Autodesk Inventor part; units mm, degrees
ref_plane "YZ Plane" through (0, 0, 0) normal (1, 0, 0) x (0, 1, 0)
ref_plane "XZ Plane" through (0, 0, 0) normal (0, 1, 0) x (-1, 0, 0)
ref_plane "XY Plane" through (0, 0, 0) normal (0, 0, 1) x (1, 0, 0)
sketch "Sketch1" plane through (0, 0, 0) normal (0, 1, 0) x (-1, 0, 0)
  circle A0 centre (0, 0) radius 10.7
  dimension "d0" = 21.4
extrude "Extrusion1" add sketch "Sketch1" along normal blind 19
sketch "Sketch2" plane through (0, 19, 0) normal (0, 1, 0) x (1, 0, 0)
  circle A0 centre (0, 0) radius 12.5
  circle A1 centre (0, 0) radius 10.7
  line L0 (-15, 8) -> (15, 8)
  line L1 (15, 8) -> (15, -8)
  line L2 (15, -8) -> (-15, -8)
  line L3 (-15, -8) -> (-15, 8)
  line L4 (0, 0) -> (1.899, 0)
  line L5 (0, 0) -> (0, 1.5989)
  point P0 (-12.5, 0)
  point P1 (9.6047, -8)
  point P2 (-9.6047, 8)
  point P3 (12.5, 0)
  point P4 (-9.6047, -8)
  point P5 (9.6047, 8)
  dimension "d9" = 25
  dimension "d10" = 21.4
  dimension "d14" = 30
  dimension "d15" = 16
extrude "Extrusion2" add sketch "Sketch2" along normal blind 5
sketch "Sketch3" plane through (0, 0, 0) normal (0, 0, 1) x (1, 0, 0)
  line L0 (10.7, 0) -> (-10.7, 0)
  line L1 (9.6047, 19) -> (15, 19)
  line L2 (15, 19) -> (15, 24)
  line L3 (-15, 24) -> (-9.6047, 24)
  line L4 (-15, 19) -> (-15, 24)
  circle A0 centre (0, 39) radius 15
  circle A1 centre (0, 39) radius 8
  line L5 (-15, 19) -> (-15, 24)
  line L6 (-15, 39) -> (-15, 24)
  line L7 (15, 39) -> (15, 24)
  line L8 (-15, 39) -> (15, 39)
  line L9 (9.6047, 24) -> (15, 24)
  line L10 (9.6047, 19) -> (9.6047, 24)
  line L11 (-15, 19) -> (-9.6047, 19)
  line L12 (-9.6047, 19) -> (-9.6047, 24)
  line L13 (-15, 24) -> (15, 24)
  point P0 (0, 0)
  point P1 (-8, 19)
  point P2 (8, 19)
  point P3 (10.7, 19)
  point P4 (-10.7, 19)
  point P5 (8, 39)
  point P6 (-8, 39)
  dimension "d16" = 30
  dimension "d17" = 30
  dimension "d18" = 16
extrude "Extrusion3" add sketch "Sketch3" along normal mid plane 16 contours L13 A0 L7 L9 | L13 L3 L6 A0 | A0 L8 A1 picked at (-12.5413, 37.8874)
sketch "Sketch4" plane through (0, 19, 0) normal (0, -1, 0) x (1, 0, 0)
  arc A0 (-9.6047, -8) -> (9.6047, -8) centre (0, 0) ccw
  line L0 (15, -8) -> (9.6047, -8)
  line L1 (15, 8) -> (15, -8)
  line L2 (9.6047, 8) -> (15, 8)
  arc A1 (9.6047, 8) -> (-9.6047, 8) centre (0, 0) ccw
  line L3 (-15, 8) -> (-9.6047, 8)
  line L4 (-15, -8) -> (-15, 8)
  line L5 (-9.6047, -8) -> (-15, -8)
  circle A2 centre (0, 0) radius 10.7
  line L6 (12.5, 5) -> (-12.5, 5)
  line L7 (-12.5, 5) -> (-12.5, -5)
  line L8 (-12.5, -5) -> (12.5, -5)
  line L9 (12.5, -5) -> (12.5, 5)
  line L10 (0, 0) -> (0, 1.5128)
  line L11 (0, 0) -> (1.2888, 0)
  dimension "d19" = 10
  dimension "d20" = 25
hole "Hole1" at (12.5, 19, 5) at (12.5, 19, -5) at (-12.5, 19, -5) at (-12.5, 19, 5) direction (0, 1, 0) diameter 3 end through all
fillet "Fillet1" radius 2 8 edges at (-15, 29, 8) (15, 29, 8) (15, 29, -8) (-15, 29, -8) (9.6047, 21.5, 8) (-9.6047, 21.5, 8) (9.6047, 21.5, -8) (-9.6047, 21.5, -8)
equation "\"d17\" = d16"
properties part number "base1" material "PVC-Piping"
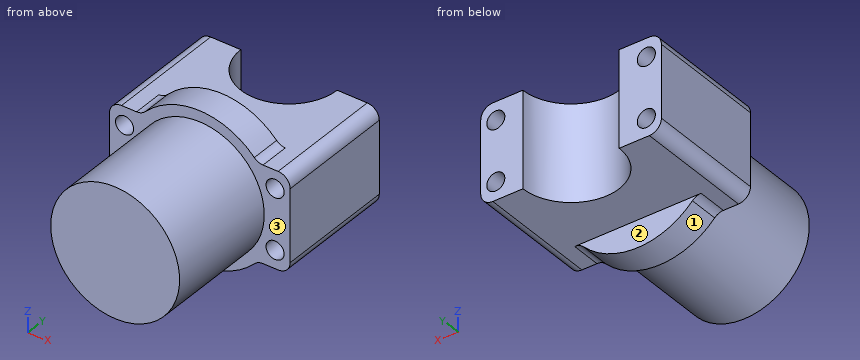
For this review, take the finished solid that the model builds, in its own axes (mm). Face numbers are marked on the shaded views. A direction names the side the tool comes from. Coordinates: 2 decimals unless noted, no trailing zeros. Loops run counter-clockwise (first coordinate to the right, second up) from the corner with the lowest first, then second, coordinate; pieces in that order, holes last.
1. Add section A-A, the plane x = -12.5. Give the boundary of the cut face in (y, z).
2. For the marked faces 1, 2 and 3, list the 3-axis set-ups (+Z, -Z, +X, -X, +Y, -Y) from which the entire face can be reached by the end or side of a thin tool; tool diameter is ignored.
3. Add section D-D, the plane y = 36.5. Give the boundary of the cut face in (x, z), then the cut area to 3 significant figures.
4. Add section B-B, the plane y = 24.5. Give the boundary of the cut face in (x, z), then the cut area to 3 significant figures.
5. Insertion check: P1, Ø2.5, axis at x = 12.5, z = 5, coming from the +Y side; P2, Ø2, axis at x = 5, y = 24.5, coming from the +Z side; P3, Ø3.5, axis at x = -5, z = 10.5, coming from the +Y side; P4, Ø1.5, axis at x = 5, y = 25.5, coming from the +Z side. Each pin has a flat end and moves straight along its axis. Give the tip position at first contact, or say it passes through.
6. Add section C-C, the plane z = 0. Give the boundary of the cut face in (x, y).
7. For line 1 (Z direction, x = -12.5, y = 29.5); line 2 (X direction, y = 33.75, z = 5); line 3 (X direction, y = 35, z = 5), list the stretches that pass through material, from the lowest coordinate up.
Result:
1. outline: (19, -8) - (39, -8) - (39, -6.5) - (19, -6.5) - close; (19, -3.5) - (39, -3.5) - (39, 3.5) - (19, 3.5) - close; (19, 6.5) - (39, 6.5) - (39, 8) - (19, 8) - close
2. face 1: -Z, +Y, -Y
2. face 2: -Z, +X, -X, +Y
2. face 3: -Y
3. outline: (-15, -6) arc R2 ccw to (-13, -8) - (-7.6, -8) - (-7.6, 8) - (-13, 8) arc R2 ccw to (-15, 6) - close; (7.6, -8) - (13, -8) arc R2 ccw to (15, -6) - (15, 6) arc R2 ccw to (13, 8) - (7.6, 8) - close; hole circle Ø3 at (-12.5, -5); hole circle Ø3 at (-12.5, 5); hole circle Ø3 at (12.5, -5); hole circle Ø3 at (12.5, 5)
3. area: 205 mm2
4. outline: (-15, -6) arc R2 ccw to (-13, -8) - (13, -8) arc R2 ccw to (15, -6) - (15, 6) arc R2 ccw to (13, 8) - (-13, 8) arc R2 ccw to (-15, 6) - close; hole circle Ø3 at (-12.5, -5); hole circle Ø3 at (-12.5, 5); hole circle Ø3 at (12.5, -5); hole circle Ø3 at (12.5, 5)
4. area: 448 mm2
5. P1: passes through
5. P2: stops at z = 11.8
5. P3: stops at y = 24
5. P4: stops at z = 8
6. outline: (-15, 19) - (-10.7, 19) - (-10.7, 0) - (10.7, 0) - (10.7, 19) - (15, 19) - (15, 39) - (8, 39) arc R8 cw to (-8, 39) - (-15, 39) - close
7. line 1: z = -8 to -6.5, -3.5 to 3.5, 6.5 to 8
7. line 2: x = -15 to -14, -11 to -6.04, 6.04 to 11, 14 to 15
7. line 3: x = -15 to -14, -11 to -6.93, 6.93 to 11, 14 to 15
